```python
from build123d import *

# Parameters (mm, degrees)
SKETCH1_W  = 154
SKETCH1_H  = 56
BASE_DEPTH = 10


with BuildPart() as part:
    # Sketch1 → base (new body)
    with BuildSketch(Plane(origin=(0, 0, 0), x_dir=(1, 0, 0), z_dir=(0, 1, 0))):
        Rectangle(SKETCH1_W, SKETCH1_H)
    extrude(amount=BASE_DEPTH)

    # Sketch4 → Cut-Revolve1 (revolve, cut)
    with BuildSketch(Plane(origin=(0, 0, 0), x_dir=(0, 0, -1), z_dir=(1, 0, 0))):
        Polygon((3, 0), (3, 2), (0, 3.732050808), (0, 0), align=None)
    revolve(axis=Axis((0, 3.732050808, 0), (0, -1, 0)), mode=Mode.SUBTRACT)


solid = part.part
```
The listing builds one solid part. Answer for the finished solid, in the listing's coordinates (mm). Coordinates: 2 decimals unless noted, no trailing zeros. Return JSON: item names as keys, results as strings. Group by question number.
Q1. For a pull along Z with two mould halves and no side action, classify faces 1 (the flat face through (-1, 5, 28)), 2 (the cylindrical face through (0, 1, 3)), 3 (the flat face through (77, 5, 0)), 4 (the conical face through (-0.468, 3.456, 0.104)) as +Z half, -Z half, draft (parallel to the pull), parting line (faces both ways), or undercut.
Q2. A flat-ended cylindrical pin translates along its axis: pin 1 Ø3.5 at (x, z) = (0, 0) entering from -Y. Find the tip coordinate at first contact, or state that the pin passes through.
Q3. Find the intervals of material crossed by line 1 along X through (y, z) = (0.6, 0), in increasing order. Write a range as [from, to].
Evaluation:
{
 "1": {"face 1": "+Z half", "face 2": "undercut", "face 3": "draft", "face 4": "undercut"},
 "2": {"pin 1": "stops at y = 2.72"},
 "3": {"line 1": "x = [-77, -3], [3, 77]"}
}
